Build history of the part. All positions in model axes, mm. A direction names the side the tool comes from. Round coordinates to 2 decimals unless told otherwise and drop trailing zeros. Loops run counter-clockwise (first coordinate to the right, second up) from the corner with the lowest first, then second, coordinate; pieces in that order, holes last. Notation, with made-up numbers: M -10.75,2 L 7.25,2 A29 ccw 7.25,40 Z; hole C 51.5,-17.75 d5. An arc over 180 degrees is marked long. One line per item, written item: value.
```python
from build123d import *

# Parameters (mm, degrees)
SKETCH1_W           = 34
SKETCH1_H           = 60
SKETCH1_R           = 0.75
BOSS_EXTRUDE1_DEPTH = 3
CHAMFER1_SIZE       = 1.3
SKETCH2_R           = 0.762
CUT_EXTRUDE1_DEPTH  = 7
SKETCH3_W           = 5
SKETCH3_H           = 4.4
CUT_EXTRUDE2_DEPTH  = 1.7
SKETCH4_R           = 0.762
CUT_EXTRUDE3_DEPTH  = 7
SKETCH5_W           = 3.3
SKETCH5_H           = 5.3
CUT_EXTRUDE4_DEPTH  = 3.5
SKETCH7_R           = 0.762
SKETCH7_W           = 7
SKETCH7_H           = 5.3
CUT_EXTRUDE5_DEPTH  = 2.5
SKETCH8_W           = 1.8
SKETCH8_H           = 17.3
CUT_EXTRUDE6_DEPTH  = 2.5
SKETCH9_R           = 3.39
CUT_EXTRUDE7_DEPTH  = 7.5
CHAMFER2_SIZE       = 3


# Some blends are built 0.0001 mm under size
with BuildPart() as part:
    # Sketch1 → Boss-Extrude1 (new body)
    with BuildSketch(Plane.XY):
        Rectangle(SKETCH1_W, SKETCH1_H)
        with Locations((-15, -21.5)):
            Circle(SKETCH1_R, mode=Mode.SUBTRACT)
        with Locations(Location((-10.5, 27.5, 0), (0, 0, 180))):
            Circle(SKETCH1_R, mode=Mode.SUBTRACT)
        with Locations((10.5, 27.5)):
            Circle(SKETCH1_R, mode=Mode.SUBTRACT)
    extrude(amount=BOSS_EXTRUDE1_DEPTH)

    # Chamfer1
    # the kernel refuses this chamfer: 1.3 mm, written as the material it takes off along each edge
    with BuildSketch(Plane(origin=(-15, -21.5, 3), x_dir=(1, 0, 0), z_dir=(0, -1, 0))) as chamfer1_piece_1:
        Polygon((0.75, -CHAMFER1_SIZE), (0.75 + CHAMFER1_SIZE, 0), (0.75, 0), align=None)
    revolve(axis=Axis((-15, -21.5, 3), (0, 0, 1)), mode=Mode.SUBTRACT)
    with BuildSketch(Plane(origin=(-10.5, 27.5, 3), x_dir=(-1, 0, 0), z_dir=(0, 1, 0))) as chamfer1_piece_2:
        Polygon((0.75, -CHAMFER1_SIZE), (0.75 + CHAMFER1_SIZE, 0), (0.75, 0), align=None)
    revolve(axis=Axis((-10.5, 27.5, 3), (0, 0, 1)), mode=Mode.SUBTRACT)
    with BuildSketch(Plane(origin=(10.5, 27.5, 3), x_dir=(1, 0, 0), z_dir=(0, -1, 0))) as chamfer1_piece_3:
        Polygon((0.75, -CHAMFER1_SIZE), (0.75 + CHAMFER1_SIZE, 0), (0.75, 0), align=None)
    revolve(axis=Axis((10.5, 27.5, 3), (0, 0, 1)), mode=Mode.SUBTRACT)

    # Sketch2 → Cut-Extrude1 (cut)
    with BuildSketch(Plane(origin=(17, 0, 0), x_dir=(0, 0, -1), z_dir=(1, 0, 0))):
        with Locations((-1.5, -21.5)):
            Circle(SKETCH2_R)
    extrude(amount=-CUT_EXTRUDE1_DEPTH, mode=Mode.SUBTRACT)

    # Sketch3 → Cut-Extrude2 (cut)
    with BuildSketch(Plane(origin=(0, 0, 0), x_dir=(-1, 0, 0), z_dir=(0, 0, -1))):
        Polygon((3.765333438, -30), (12, -30), (12, -24.8), (7, -24.8), (3.765333438, -24.8), align=None)
        with Locations((9.5, -22.6)):
            Rectangle(SKETCH3_W, SKETCH3_H)
    extrude(amount=-CUT_EXTRUDE2_DEPTH, mode=Mode.SUBTRACT)

    # Sketch4 → Cut-Extrude3 (cut)
    with BuildSketch(Plane.XZ.offset(30)):
        with Locations(Location((15, 1.5, 0), (0, 0, 270))):
            Circle(SKETCH4_R)
    extrude(amount=-CUT_EXTRUDE3_DEPTH, mode=Mode.SUBTRACT)

    # Sketch5 → Cut-Extrude4 (cut)
    with BuildSketch(Plane(origin=(0, 0, 0), x_dir=(-1, 0, 0), z_dir=(0, 0, -1))):
        with Locations((-3, 7.425)):
            Rectangle(SKETCH5_W, SKETCH5_H)
    extrude(amount=-CUT_EXTRUDE4_DEPTH, mode=Mode.SUBTRACT)

    # Sketch7 → Cut-Extrude5 (cut)
    with BuildSketch(Plane(origin=(0, 0, 0), x_dir=(-1, 0, 0), z_dir=(0, 0, -1))):
        with Locations((-13.25, 17.75)):
            Circle(SKETCH7_R)
        with Locations((7.25, 17.75)):
            Circle(SKETCH7_R)
        with Locations(Location((7.25, -2.9, 0), (0, 0, 180))):
            Circle(SKETCH7_R)
        with Locations(Location((-13.25, -2.9, 0), (0, 0, 180))):
            Circle(SKETCH7_R)
        with Locations((-3, 17.2)):
            Rectangle(SKETCH7_W, SKETCH7_H)
        with Locations((-3, -2.35)):
            Rectangle(SKETCH7_W, SKETCH7_H)
    extrude(amount=-CUT_EXTRUDE5_DEPTH, mode=Mode.SUBTRACT)

    # Sketch8 → Cut-Extrude6 (cut)
    with BuildSketch(Plane(origin=(0, 0, 0), x_dir=(-1, 0, 0), z_dir=(0, 0, -1))):
        with Locations((8.8, 7.53)):
            Rectangle(SKETCH8_W, SKETCH8_H)
        with Locations((-14.8, 7.53)):
            Rectangle(SKETCH8_W, SKETCH8_H)
    extrude(amount=-CUT_EXTRUDE6_DEPTH, mode=Mode.SUBTRACT)

    # Sketch9 → Cut-Extrude7 (cut)
    with BuildSketch(Plane(origin=(0, 0, 0), x_dir=(-1, 0, 0), z_dir=(0, 0, -1))):
        with Locations((-1, -10.79)):
            Circle(SKETCH9_R)
    extrude(amount=-CUT_EXTRUDE7_DEPTH, mode=Mode.SUBTRACT)

    # Chamfer2
    chamfer2_edges = [part.edges().sort_by_distance(p)[0] for p in [
        (4.65, 7.425, 3),
        (3, 4.775, 3),
        (1.35, 7.425, 3),
        (3, 10.075, 3),
    ]]
    chamfer(chamfer2_edges, length=CHAMFER2_SIZE - 0.0001)  # a hair under: the kernel refuses the full size


solid = part.part
```
Item 1: Slice it at B-B, the plane y = 27.5. Give the cut face in (x, z).
Check values:
outline: M -17,0 L -11.25,0 L -11.25,1.7 L -12.55,3 L -17,3 Z; M -9.75,0 L 9.75,0 L 9.75,1.7 L 8.45,3 L -8.45,3 L -9.75,1.7 Z; M 11.25,0 L 17,0 L 17,3 L 12.55,3 L 11.25,1.7 Z
Item 2: Slice it at C-C, the plane x = 15. Give the cut face in (y, z).
Check values:
outline: M -30,0 L -1.12,0 L -1.12,2.5 L 16.18,2.5 L 16.18,0 L 30,0 L 30,3 L -30,3 L -30,2.26 L -23,2.26 L -23,0.74 L -30,0.74 Z; hole C -21.5,1.5 d1.52
Item 3: Wall check: line 1 along Y through (x, z) = (-7.25, 0.65); line 2 along X through (y, z) = (-2.9, 2); line 3 along Y through (x, z) = (-15, 0.7). Give the ranges that are in metal, low to high.
Check values:
line 1: y = -20.4 to -3.66, -2.14 to 16.99, 18.51 to 30
line 2: x = -17 to -8.01, -6.49 to -0.5, 6.5 to 12.49, 14.01 to 17
line 3: y = -30 to -22.25, -20.75 to 30
Item 4: Drop flat-ended pins along their axis: P1, Ø1.5, axis at x = 1.5, y = 18.5, coming from the -Z side; P2, Ø0.8, axis at x = -5, z = 1, coming from the -Y side. Give the stop position or say it passes through.
Check values:
P1: stops at z = 2.5
P2: stops at y = -24.8
Item 5: Slice it at A-A, the plane x = -10.5. Give the cut face in (y, z), and give its area (3 significant figures).
Check values:
outline: M -30,1.7 L -20.4,1.7 L -20.4,0 L 26.75,0 L 26.75,1.7 L 25.45,3 L -30,3 Z; M 28.25,0 L 30,0 L 30,3 L 29.55,3 L 28.25,1.7 Z
area: 157 mm2
Item 6: Pull direction X, two halves, no side cores. Call faces 1 (the face through (14.01, 17.78, 1.23)), 2 (the face through (-17, 0, 1)), 3 (the face through (17, 0, 1)): pulls with the +X half, pulls with the -X half, needs draft (parallel to the pull), parting line crosses it, or undercut.
Check values:
face 1: undercut
face 2: pulls with the -X half
face 3: pulls with the +X half
Item 7: Which spindle directions (+Z, -Z, +X, -X, +Y, -Y) get a long thin tool onto all of the face, cutting with end or side? Do faces 4 (the face through (13, 18, 2.5)), 5 (the face through (15.756, -26.549, 1.599)), 6 (the face through (-7, -23, 1)), 7 (the face through (-0.46, 7.5, 1.81)). Say none if no direction does.
Check values:
face 4: -Z
face 5: -Y
face 6: -Z, -Y
face 7: +Z
